CAD build for the part. Positions are in the model's coordinates, mm. Give positions to 0.01 mm unless a question says otherwise; leave off trailing zeros. Loops run counter-clockwise (first coordinate to the right, second up) from the corner with the lowest first, then second, coordinate; pieces in that order, holes last. Notation, with made-up numbers: (59.25, 35.5) - (82.25, 35.5) arc R20 ccw to (82.25, 48.5) - close; hole circle Ø8 at (-32.75, 36.25). An arc over 180 degrees is marked (long way). Return JSON: item names as keys, results as strings.
Autodesk Inventor part; units mm, degrees
ref_plane "YZ Plane" through (0, 0, 0) normal (1, 0, 0) x (0, 1, 0)
ref_plane "XZ Plane" through (0, 0, 0) normal (0, 1, 0) x (-1, 0, 0)
ref_plane "XY Plane" through (0, 0, 0) normal (0, 0, 1) x (1, 0, 0)
sketch "Sketch1" plane through (0, 0, 0) normal (0, 1, 0) x (-1, 0, 0)
  circle A0 centre (0, -18) radius 1.55
  circle A1 centre (0, 18) radius 1.55
  line L0 (0, 25) -> (0, 25)
  line L1 (-5, 20) -> (-5, -20)
  line L2 (0, -25) -> (0, -25)
  line L3 (5, -20) -> (5, 20)
  arc A2 (5, 20) -> (0, 25) centre (0, 20) ccw
  arc A3 (0, 25) -> (-5, 20) centre (0, 20) ccw
  arc A4 (-5, -20) -> (0, -25) centre (0, -20) ccw
  arc A5 (0, -25) -> (5, -20) centre (0, -20) ccw
  point P0 (0, 0)
  point P1 (-5, -25)
  point P2 (-5, 25)
  point P3 (5, -25)
  point P4 (0, -25)
  dimension "d0" = 3.1
  dimension "d1" = 3.1
  dimension "d2" = 10
  dimension "d3" = 50
  dimension "d4" = 5
extrude "Extrusion1" add sketch "Sketch1" along normal blind 1.25
properties part number "KreplenieBoltam" material "Iron, Cast"
1. Pull direction X, two halves, no side cores. Call faces 1 (the face through (5, 1, 0)), 2 (the face through (0.202, 0.616, 16.463)), 3 (the face through (0, 1, 25)), 4 (the face through (0.202, 0.616, -19.537)): +X half, -X half, draft (parallel to the pull), parting line (faces both ways), or undercut.
Values follow:
{"face 1": "+X half", "face 2": "undercut", "face 3": "parting line", "face 4": "undercut"}
2. Cut at B-B, the plane x = 0. Write the cut outline in (y, z).
Values follow:
{"outline": "(0, -25) - (1.25, -25) - (1.25, -19.55) - (0, -19.55) - close; (0, -16.45) - (1.25, -16.45) - (1.25, 16.45) - (0, 16.45) - close; (0, 19.55) - (1.25, 19.55) - (1.25, 25) - (0, 25) - close"}
3. Cut at C-C, the plane y = 0.7. Write the cut outline in (x, z), plus the area to 3 significant figures.
Values follow:
{"outline": "(-5, -20) arc R5 ccw to (5, -20) - (5, 20) arc R5 ccw to (-5, 20) - close; hole circle Ø3.1 at (0, -18); hole circle Ø3.1 at (0, 18)", "area": "463 mm²"}
4. Cut at A-A, the plane z = -18. Write the cut outline in (x, y), plus the area to 4 significant figures.
Values follow:
{"outline": "(-5, 0) - (-1.55, 0) - (-1.55, 1.25) - (-5, 1.25) - close; (1.55, 0) - (5, 0) - (5, 1.25) - (1.55, 1.25) - close", "area": "8.625 mm²"}
5. Cut at D-D, the plane x = -4. Write the cut outline in (y, z).
Values follow:
{"outline": "(0, -23) - (1.25, -23) - (1.25, 23) - (0, 23) - close"}
6. Drill centre lines: probe 1 along Z at (x, y) = (0, 0.95); probe 2 along Z at (x, y) = (0.75, 0.65); probe 3 along Z at (x, y) = (-2.75, 0.95). Where is each one in solid material? Low to high.
Values follow:
{"probe 1": "z = -25 to -19.55, -16.45 to 16.45, 19.55 to 25", "probe 2": "z = -24.94 to -19.36, -16.64 to 16.64, 19.36 to 24.94", "probe 3": "z = -24.18 to 24.18"}
7. Drop a flat-ended pin along its axis: P1, Ø5, axis at x = 0, z = 18, coming from the +Y side. Give the stop position or say it passes through.
Values follow:
{"P1": "stops at y = 1.25"}
